Autodesk Fusion 360 part; units mm, degrees
sketch "Sketch1" plane through (0, 0, 0) normal (0, 0, 1) x (1, 0, 0)
  line L0 (0, 0) -> (36, 0)
  line L1 (36, 0) -> (36, 18)
  line L2 (36, 18) -> (0, 18)
  line L3 (0, 18) -> (0, 0)
  dimension "d1" = 36
  dimension "d2" = 18
extrude "Extrude1" add sketch "Sketch1" along normal blind 20
sketch "Sketch2" plane through (0, 0, 20) normal (0, 0, 1) x (-1, 0, 0)
  line L0 (0, -18) -> (0, 0)
  line L1 (0, 0) -> (-36, 0)
  line L2 (-36, 0) -> (-36, -18)
  line L3 (-36, -18) -> (0, -18)
  circle A0 centre (-18, -18) radius 13
  dimension "d5" = 26
extrude "Extrude2" cut sketch "Sketch2" against normal blind 20 contours L3 A0 picked at (-19.0768, -11.2377)
ref_plane "WorkPlane1" through (0, 20, 0) normal (0, 1, 0) x (0, 0, 1)
sketch "Sketch7" plane through (0, 0, 0) normal (0, -1, 0) x (1, 0, 0)
  line L0 (0, 0) -> (36, 0)
  line L1 (36, 20) -> (0, 20)
  line L2 (0, 20) -> (0, 0)
  line L3 (18, 10) -> (18, 23) construction
  line L4 (36, 0) -> (36, 20)
sketch "Sketch6" plane through (36, 0, 0) normal (1, 0, 0) x (0, 1, 0)
  line L0 (0, 0) -> (18, 0)
  line L1 (18, 0) -> (18, 20)
  line L2 (18, 20) -> (0, 20)
  line L3 (0, 20) -> (0, 0)
  line L4 (0, 20) -> (18, 0) construction
  line L5 (0, 0) -> (18, 20) construction
  line L6 (9, 10) -> (18, 10) construction
  line L7 (9, 10) -> (9, 0) construction
  line L8 (9, 10) -> (9, 20) construction
  line L9 (13.5, 17.5) -> (18, 17.5) construction
  line L10 (13.5, 5) -> (13.5, 10) construction
  line L11 (18, 7.5) -> (18, 12.5311)
  line L12 (13.5, 17.5) -> (18, 17.5)
  line L13 (18, 17.5) -> (18, 2.5)
  line L14 (18, 2.5) -> (13.5, 2.5)
  line L15 (13.5, 2.5) -> (13.5, 17.5)
  dimension "d25" = 15
  dimension "d26" = 4.5
  dimension "d34" = 7.5
extrude "Extrude7" add sketch "Sketch6" along normal blind 8 contours L1 L11 L12 L13 L14 L15
sketch "Sketch11" plane through (0, 13.5, 0) normal (0, -1, 0) x (1, 0, 0)
  line L0 (36, 17.5) -> (36, 2.5)
  line L1 (36, 2.5) -> (44, 2.5)
  line L2 (44, 2.5) -> (44, 17.5)
  line L3 (44, 17.5) -> (36, 17.5)
  circle A0 centre (40, 13) radius 1.1
  circle A1 centre (40, 7) radius 1.1
  line L4 (36, 0) -> (36, 20)
  line L5 (36, 20) -> (0, 20)
  line L6 (18, 10) -> (18, 23)
  circle A2 centre (-4, 13) radius 1.1
  circle A3 centre (-4, 7) radius 1.1
  dimension "d30" = 2.2
  dimension "d31" = 2.2
  dimension "d35" = 6
  dimension "d36" = 4
  dimension "d37" = 4
  dimension "d38" = 7
sketch "Sketch12" plane through (0, 0, 0) normal (-1, 0, 0) x (0, -1, 0)
  line L0 (-18, 0) -> (0, 0)
  line L1 (0, 0) -> (0, 20)
  line L2 (0, 20) -> (-18, 20)
  line L3 (-18, 20) -> (-18, 0)
  line L4 (-18, 17.5) -> (-13.5, 17.5)
  line L5 (-13.5, 17.5) -> (-13.5, 2.5)
  line L6 (-13.5, 2.5) -> (-18, 2.5)
  line L7 (-18, 2.5) -> (-18, 17.5)
  line L8 (-18, 10) -> (-8, 10) construction
  dimension "d39" = 15
  dimension "d40" = 7.5
  dimension "d41" = 4.5
extrude "Extrude8" add sketch "Sketch12" along normal blind 8 contours L3 L4 L5 L6 L7
extrude "Extrude9" cut sketch "Sketch11" against normal blind 4.5 contours A0 | A1 | A2 | A3
sketch "Sketch13" plane through (0, 0, 20) normal (0, 0, 1) x (-1, 0, 0)
  arc A0 (-5, -18) -> (-31, -18) centre (-18, -18) ccw
  line L0 (-5, -18) -> (0, -18)
  line L1 (0, -18) -> (0, 0)
  line L2 (0, 0) -> (-36, 0)
  line L3 (-36, 0) -> (-36, -18)
  line L4 (-36, -18) -> (-31, -18)
  line L5 (-34.8, -18) -> (-34.8, 0) construction
  dimension "d46" = 3.8
sketch "Sketch14" plane through (18, 0, 10) normal (0, -1, 0) x (1, 0, 0)
  line L0 (16.8, 10) -> (13.8, 10)
  line L1 (13.8, 10) -> (13.8, 0)
  line L2 (13.8, 0) -> (16.8, 0)
  line L3 (16.8, 0) -> (16.8, 10)
  point P0 (16.8, 10)
  dimension "d47" = 3
  dimension "d48" = 10
extrude "Extrude10" add sketch "Sketch14" along normal blind 14.8
sketch "Sketch15" plane through (34.8, 0, 0) normal (1, 0, 0) x (0, 1, 0)
  line L0 (0, 10) -> (0, 20)
  line L1 (0, 20) -> (-14.8, 20)
  line L2 (-14.8, 20) -> (-14.8, 10)
  line L3 (-14.8, 10) -> (0, 10)
  circle A0 centre (-8.4, 15) radius 3.1
  dimension "d51" = 6.2
  dimension "d52" = 6.4
  dimension "d53" = 5
extrude "Extrude11" cut sketch "Sketch15" against normal blind 3 contours A0
fillet "Fillet1" radius 5 2 edges at (33.3, -14.8, 20) (33.3, -14.8, 10)
fillet "Fillet2" radius 2 1 edges at (36, 0, 10)
fillet "Fillet3" radius 12 1 edges at (0, 0, 10)
fillet "Fillet4" radius 0.5 1 edges at (0, 13.5, 10)
fillet "Fillet5" radius 1 2 edges at (-8, 18, 10) (-8, 13.5, 10)
fillet "Fillet6" radius 1 2 edges at (44, 13.5, 10) (44, 18, 10)
fillet "Fillet7" radius 0.5 1 edges at (36, 13.5, 10)
fillet "Fillet8" radius 0.5 1 edges at (31.8, 0, 15)
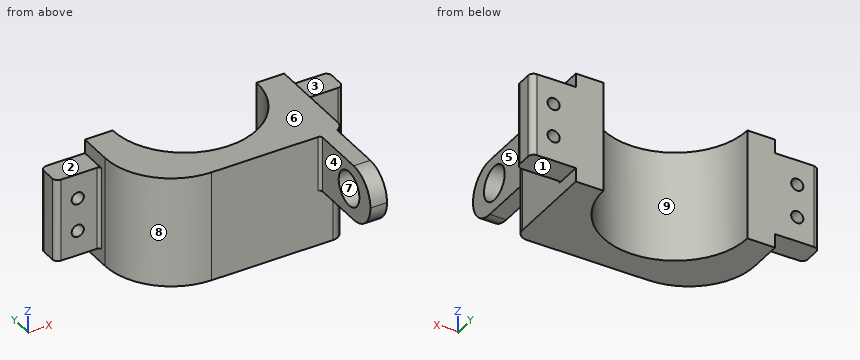
Geometry: final body of the model. Coordinates: model frame, mm. Face numbers are marked on the shaded views. A direction names the side the tool comes from. Give positions to 0.01 mm unless a question says otherwise; leave off trailing zeros. Write each loop counter-clockwise with the first axis right and the second up, starting at its lowest first coordinate (ties: lowest second). Pieces come first, ordered by that corner, then holes.
(1) Access query for the marked faces 1, 2, 3, 4 and 5. Directions: +Z, -Z, +X, -X, +Y, -Y. A direction counts if a zero-diameter tool reaches every point of the face in a straight line with its end or side. Return the directions, or none.
(2) Mould query, pull axis Y, two halves, no side actions, for the marked faces 6, 7, 8 and 9. Classes: released by +Y, released by -Y, zero draft, split by the parting line, or undercut.
(3) Cut plane D-D, the plane x = 18. Return loops of the section in (y, z), then the cut area to 3 significant figures.
(4) Cut plane B-B, the plane x = -4. Return loops of the section in (y, z), then the cut area to 3 significant figures.
(5) Cut plane C-C, the plane z = 13. Give the number of separate pieces and of enclosed holes in the cut face, then the cut area to 3 significant figures.
(6) Cut plane A-A, the plane z = 7. Return loops of the section in (x, y).
(7) Ray query, line 1 (Z direction, x = 40, y = 15); line 2 (Y direction, x = 38.5, z = 5.75); line 3 (Z direction, x = 39, y = 16). Return the intervals inside material, ascending.
(8) First-contact query: P1, Ø7, axis at y = -8.4, z = 15, coming from the -X side; P2, Ø5.5, axis at x = -3.5, y = 14.5, coming from the +Z side; P3, Ø7, axis at x = -4.5, z = 9, coming from the -Y side; P4, Ø10, axis at y = 10, z = 12, coming from the -X side. Flat tips, straight axial feed; report the tip coordinate or a pass-through.
Values follow:
1. face 1: -Z, +X, +Y, -Y
1. face 2: +Z, -X, +Y, -Y
1. face 3: +Z, +X, +Y, -Y
1. face 4: +Z, -Z, -X, -Y
1. face 5: +Z, -Z, +X, -Y
2. face 6: zero draft
2. face 7: undercut
2. face 8: released by -Y
2. face 9: released by +Y
3. outline: (0, 0) - (5, 0) - (5, 20) - (0, 20) - close
3. area: 100 mm2
4. outline: (13.5, 2.5) - (18, 2.5) - (18, 5.9) - (13.5, 5.9) - close; (13.5, 8.1) - (18, 8.1) - (18, 11.9) - (13.5, 11.9) - close; (13.5, 14.1) - (18, 14.1) - (18, 17.5) - (13.5, 17.5) - close
4. area: 47.7 mm2
5. separate pieces: 4
5. enclosed holes: 0
5. area: 431 mm2
6. outline: (-8, 14.5) arc R1 ccw to (-7, 13.5) - (-5.1, 13.5) - (-5.1, 18) - (-7, 18) arc R1 ccw to (-8, 17) - close; (-2.9, 13.5) - (-0.5, 13.5) arc R0.5 cw to (0, 13) - (0, 12) arc R12 ccw to (12, 0) - (34, 0) arc R2 ccw to (36, 2) - (36, 13) arc R0.5 cw to (36.5, 13.5) - (38.9, 13.5) - (38.9, 18) - (31, 18) arc R13 cw to (5, 18) - (-2.9, 18) - close; (41.1, 13.5) - (43, 13.5) arc R1 ccw to (44, 14.5) - (44, 17) arc R1 ccw to (43, 18) - (41.1, 18) - close
7. line 1: z = 2.5 to 5.9, 8.1 to 11.9, 14.1 to 17.5
7. line 2: y = 13.5 to 18
7. line 3: z = 2.5 to 6.54, 7.46 to 12.54, 13.46 to 17.5
8. P1: stops at x = 31.8
8. P2: stops at z = 17.5
8. P3: stops at y = 13.5
8. P4: stops at x = -8
